Design review of the part shown in the three views and the two pictorial views. Dimensions are in mm from the part's minimum x, y and z. A direction names the side the tool comes from. Coordinates: 2 decimals unless noted, no trailing zeros. Write each loop counter-clockwise with the first axis right and the second up, starting at its lowest first coordinate (ties: lowest second). Pieces come first, ordered by that corner, then holes.
Q1. For the marked faces 1 and 2, list the 3-axis set-ups (+Z, -Z, +X, -X, +Y, -Y) from which the entire face can be reached by the end or side of a thin tool; tool diameter is ignored.
Q2. Take a section at A-A, the plane y = 0.7. Write out the cut boundary in (x, z).
Q3. Take a section at C-C, the plane z = 3.25. Write out the cut boundary in (x, y).
Q4. For L1, parallel to Z at x = 3.5, y = 0.85; L2, parallel to Z at x = 4.25, y = 0.95 (1 decimal); L3, parallel to Y at x = 3.25, z = 6.5, list the stretches that pass through material, from the lowest coordinate up.
Q5. The part is to be moulded in two halves that separate along X. For the marked faces 3, 4 and 5, say which applies: released by +X, released by -X, zero draft, split by the parting line, or undercut.
Q6. Take a section at B-B, the plane x = 1.25. Write out the cut boundary in (y, z).
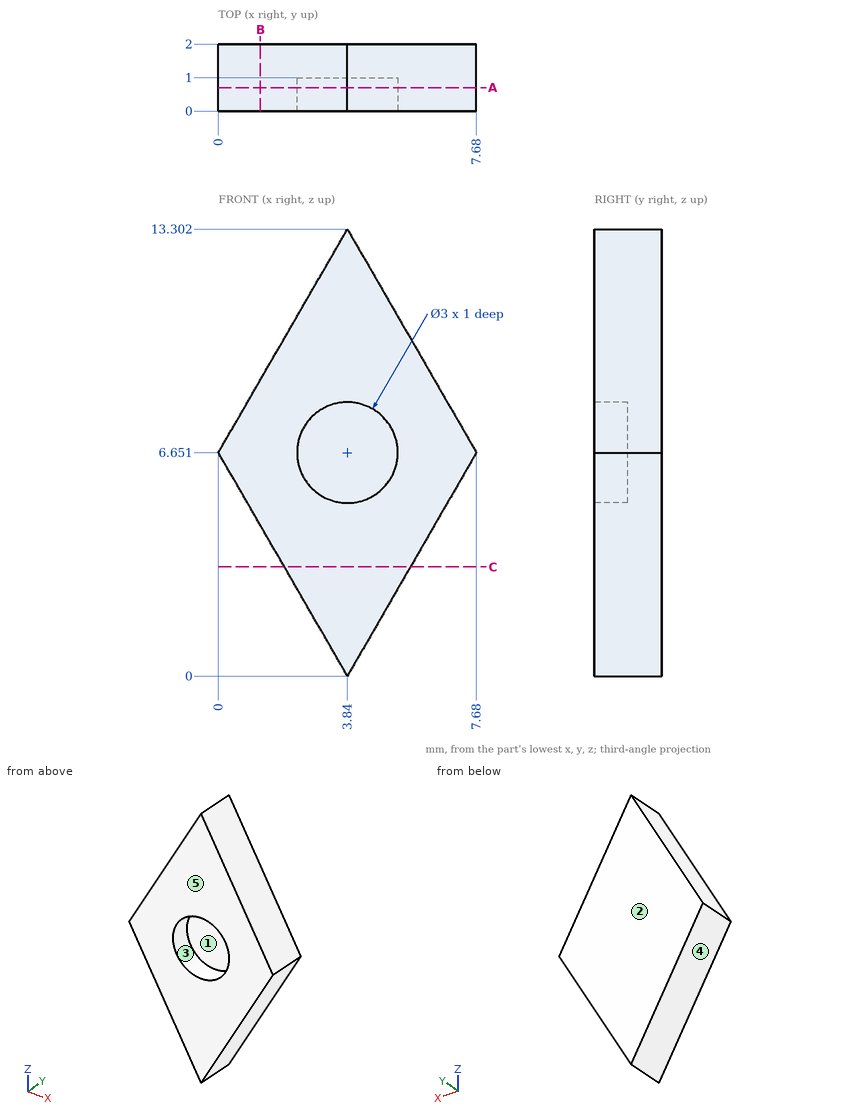
Responses:
1. face 1: -Y
1. face 2: +Z, -Z, +X, -X, +Y
2. outline: (0, 6.65) - (3.84, 0) - (7.68, 6.65) - (3.84, 13.3) - close; hole circle Ø3 at (3.84, 6.65)
3. outline: (1.96, 0) - (5.72, 0) - (5.72, 2) - (1.96, 2) - close
4. L1: z = 0.59 to 5.19, 8.11 to 12.71
4. L2: z = 0.7 to 5.2, 8.1 to 12.6
4. L3: y = 1 to 2
5. face 3: undercut
5. face 4: released by -X
5. face 5: zero draft
6. outline: (0, 4.49) - (2, 4.49) - (2, 8.82) - (0, 8.82) - close
